Source: CAD feature listing. Evaluate the final solid. Frame: model axes, mm. A direction names the side the tool comes from. Coordinates: 2 decimals unless noted, no trailing zeros. Write each loop counter-clockwise with the first axis right and the second up, starting at its lowest first coordinate (ties: lowest second). Pieces come first, ordered by that corner, then holes. Notation, with made-up numbers: (61.25, -15.75) -> (68.25, -15.75) arc R26 cw to (68.25, 7.25) -> close; hole circle Ø4 at (-2, 22). An arc over 180 degrees is marked (long way). Write item = value, one per line.
from build123d import *

# Parameters (mm, degrees)
SKETCH1_R           = 31.55
BOSS_EXTRUDE1_DEPTH = 10
SKETCH3_R           = 4.15
CUT_EXTRUDE1_DEPTH  = 10
SKETCH5_R           = 31.55
SKETCH5_R_2         = 28.75
BOSS_EXTRUDE2_DEPTH = 50


with BuildPart() as part:
    # Sketch1 → Boss-Extrude1 (new body)
    with BuildSketch(Plane(origin=(0, 0, 0), x_dir=(1, 0, 0), z_dir=(0, 1, 0))):
        with Locations(Location((0, 0, 0), (0, 0, 270))):
            Circle(SKETCH1_R)
    extrude(amount=BOSS_EXTRUDE1_DEPTH)

    # Sketch3 → Cut-Extrude1 (cut)
    with BuildSketch(Plane(origin=(0, 10, 0), x_dir=(1, 0, 0), z_dir=(0, 1, 0))):
        with Locations(Location((-18.765, 0, 0), (0, 0, 270))):
            Circle(SKETCH3_R)
        with Locations(Location((18.765, 0, 0), (0, 0, 270))):
            Circle(SKETCH3_R)
    extrude(amount=-CUT_EXTRUDE1_DEPTH, mode=Mode.SUBTRACT)

    # Sketch5 → Boss-Extrude2 (add)
    with BuildSketch(Plane(origin=(0, 10, 0), x_dir=(1, 0, 0), z_dir=(0, 1, 0))):
        with Locations(Location((0, 0, 0), (0, 0, 270))):
            Circle(SKETCH5_R)
        with Locations(Location((0, 0, 0), (0, 0, 270))):
            Circle(SKETCH5_R_2, mode=Mode.SUBTRACT)
    extrude(amount=BOSS_EXTRUDE2_DEPTH)


solid = part.part
1) Pull-direction query (Z, two-part tool) for faces 3 (the flat face through (0, 0, 0)), 4 (the flat face through (0, 10, 0)), 5 (the cylindrical face through (-19.198, 29.58, -25.037)); classes: +Z half, -Z half, draft (parallel to the pull), parting line (faces both ways), or undercut.
Answer block:
face_3 = draft
face_4 = undercut
face_5 = parting line
2) First-contact query: pin 1 Ø3 at (y, z) = (50, 21) entering from +X; pin 2 Ø8 at (y, z) = (7, -16.5) entering from +X; pin 3 Ø6 at (x, z) = (-15, 13) entering from -Y; pin 4 Ø2 at (x, y) = (-23, 9.5) entering from +Z. Flat tips, straight axial feed; report the tip coordinate or a pass-through.
Answer block:
pin_1 = 24.8
pin_2 = 28.97
pin_3 = 0
pin_4 = 22.61
3) Cut plane A-A, the plane z = 0. Output: boundary loops of the cut face in (x, y) (3 decimals), and give its area (3 significant figures).
Answer block:
outline = (-31.55, 0) -> (-22.915, 0) -> (-22.915, 10) -> (-28.75, 10) -> (-28.75, 60) -> (-31.55, 60) -> close; (-14.615, 0) -> (14.615, 0) -> (14.615, 10) -> (-14.615, 10) -> close; (22.915, 0) -> (31.55, 0) -> (31.55, 60) -> (28.75, 60) -> (28.75, 10) -> (22.915, 10) -> close
area = 745 mm2
4) Cut plane D-D, the plane y = 53. Output: boundary loops of the cut face in (x, z), and give its area (3 significant figures).
Answer block:
outline = circle Ø63.1 at (0, 0); hole circle Ø57.5 at (0, 0)
area = 530 mm2
5) Material intervals for probe 1 along X at (y, z) = (6.75, 0) (3 decimals); probe 2 along X at (y, z) = (47.5, 0); probe 3 along Z at (x, y) = (16, 50), sorted ascending. Write a range as [from, to].
Answer block:
probe_1 = [-31.55, -22.915], [-14.615, 14.615], [22.915, 31.55]
probe_2 = [-31.55, -28.75], [28.75, 31.55]
probe_3 = [-27.19, -23.89], [23.89, 27.19]
6) Cut plane B-B, the plane x = -22. Output: boundary loops of the cut face in (y, z), and give its area (3 significant figures).
Answer block:
outline = (0, -22.61) -> (60, -22.61) -> (60, -18.51) -> (10, -18.51) -> (10, -2.6) -> (0, -2.6) -> close; (0, 2.6) -> (10, 2.6) -> (10, 18.51) -> (60, 18.51) -> (60, 22.61) -> (0, 22.61) -> close
area = 811 mm2
7) Reachability of faces 1 (the cylindrical face through (22.88, 5.07, -0.54)), 2 (the cylindrical face through (-28.066, 34.65, -6.232)) from +Z, -Z, +X, -X, +Y, -Y: full face, straight path, thin tool, end or side. Return the list, or none.
Answer block:
face_1 = +Y, -Y
face_2 = +Y
8) Cut plane C-C, the plane x = 0. Output: boundary loops of the cut face in (y, z), and give its area (3 significant figures).
Answer block:
outline = (0, -31.55) -> (60, -31.55) -> (60, -28.75) -> (10, -28.75) -> (10, 28.75) -> (60, 28.75) -> (60, 31.55) -> (0, 31.55) -> close
area = 911 mm2
